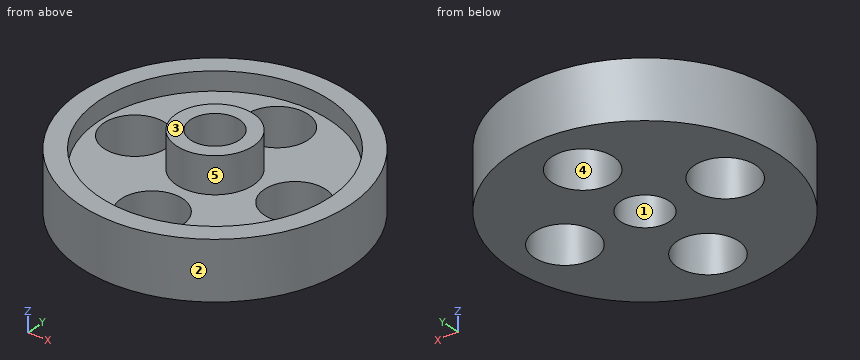
from build123d import *

# Parameters (mm, degrees)
F0_R     = 35.0012
F0_R_2   = 29.9974
F1_DEPTH = 15.0114
F0_R_3   = 8.001
F0_R_4   = 9.9949
F2_DEPTH = 10.16
F0_R_5   = 6.3373
F3_DEPTH = 19.5072


# Not quite as in the source:
# - a feature names something its author has since deleted; it is built from what else it names


with BuildPart() as f1:
    # F0 (on Top) → F1 (new body)
    with BuildSketch(Plane.XY):
        Circle(F0_R)
        Circle(F0_R_2, mode=Mode.SUBTRACT)
    extrude(amount=F1_DEPTH)

    # F0 (on Top) → F2 (join)
    with BuildSketch(Plane.XY):
        Circle(F0_R_2)
        with Locations((0.1067890262, -20.8610873669)):
            Circle(F0_R_3, mode=Mode.SUBTRACT)
        with Locations((20.7458101213, -0.0499814087)):
            Circle(F0_R_3, mode=Mode.SUBTRACT)
        with Locations((-20.7319166511, 0)):
            Circle(F0_R_3, mode=Mode.SUBTRACT)
        Circle(F0_R_4, mode=Mode.SUBTRACT)
        with Locations((0, 20.5026287585)):
            Circle(F0_R_3, mode=Mode.SUBTRACT)
    extrude(amount=F2_DEPTH)

    # F0 (on Top) → F3 (join)
    with BuildSketch(Plane.XY):
        Circle(F0_R_4)
        Circle(F0_R_5, mode=Mode.SUBTRACT)
    extrude(amount=F3_DEPTH)


solid = f1.part
Geometry: final body of the model. Coordinates: model frame, mm. Face numbers are marked on the shaded views. A direction names the side the tool comes from. Give positions to 0.01 mm unless a question says otherwise; leave off trailing zeros. Write each loop counter-clockwise with the first axis right and the second up, starting at its lowest first coordinate (ties: lowest second). Pieces come first, ordered by that corner, then holes.
(1) First-contact query: P1, Ø6, axis at x = -8.5, z = 12.5, coming from the -Y side; P2, Ø10, axis at y = 18, z = 13.5, coming from the -X side; P3, Ø2, axis at y = 7, z = 3, coming from the -X side. Flat tips, straight axial feed; report the tip coordinate or a pass-through.
(2) Cut plane D-D, the plane y = -4.5. Return loops of the section in (x, z).
(3) Ray query, line 1 (Y direction, x = 8.5, z = 11); line 2 (Y direction, x = 0, z = 13.2); line 3 (X direction, y = -4, z = 12). Return the intervals inside material, ascending.
(4) Mould query, pull axis Y, two halves, no side actions, for the marked faces 1, 2 and 3. Classes: released by +Y, released by -Y, zero draft, split by the parting line, or undercut.
(5) Cut plane A-A, the plane x = -14.5. Return loops of the section in (y, z).
(6) Access query for the marked faces 4 and 5. Directions: +Z, -Z, +X, -X, +Y, -Y. A direction counts if a zero-diameter tool reaches every point of the face in a straight line with its end or side. Return the directions, or none.
(7) Cut plane B-B, the plane x = 0. Return loops of the section in (y, z).
(8) Cut plane C-C, the plane y = -16.5. Return loops of the section in (x, z), then the cut area to 3 significant figures.
Values follow:
1. P1: stops at y = -34.57
1. P2: stops at x = -32.5
1. P3: stops at x = -34.48
2. outline: (-34.71, 0) - (-27.35, 0) - (-27.35, 10.16) - (-29.66, 10.16) - (-29.66, 15.01) - (-34.71, 15.01) - close; (-14.12, 0) - (-4.46, 0) - (-4.46, 19.51) - (-8.92, 19.51) - (-8.92, 10.16) - (-14.12, 10.16) - close; (4.46, 0) - (14.1, 0) - (14.1, 10.16) - (8.92, 10.16) - (8.92, 19.51) - (4.46, 19.51) - close; (27.4, 0) - (34.71, 0) - (34.71, 15.01) - (29.66, 15.01) - (29.66, 10.16) - (27.4, 10.16) - close
3. line 1: y = -33.95 to -28.77, -5.26 to 5.26, 28.77 to 33.95
3. line 2: y = -35 to -30, -9.99 to -6.34, 6.34 to 9.99, 30 to 35
3. line 3: x = -34.77 to -29.73, -9.16 to -4.92, 4.92 to 9.16, 29.73 to 34.77
4. face 1: undercut
4. face 2: split by the parting line
4. face 3: zero draft
5. outline: (-31.86, 0) - (-5.02, 0) - (-5.02, 10.16) - (-26.26, 10.16) - (-26.26, 15.01) - (-31.86, 15.01) - close; (5.02, 0) - (31.86, 0) - (31.86, 15.01) - (26.26, 15.01) - (26.26, 10.16) - (5.02, 10.16) - close
6. face 4: +Z, -Z
6. face 5: +Z
7. outline: (-35, 0) - (-28.86, 0) - (-28.86, 10.16) - (-30, 10.16) - (-30, 15.01) - (-35, 15.01) - close; (-12.86, 0) - (-6.34, 0) - (-6.34, 19.51) - (-9.99, 19.51) - (-9.99, 10.16) - (-12.86, 10.16) - close; (6.34, 0) - (12.5, 0) - (12.5, 10.16) - (9.99, 10.16) - (9.99, 19.51) - (6.34, 19.51) - close; (28.5, 0) - (35, 0) - (35, 15.01) - (30, 15.01) - (30, 10.16) - (28.5, 10.16) - close
8. outline: (-30.87, 0) - (-6.6, 0) - (-6.6, 10.16) - (-25.05, 10.16) - (-25.05, 15.01) - (-30.87, 15.01) - close; (6.81, 0) - (30.87, 0) - (30.87, 15.01) - (25.05, 15.01) - (25.05, 10.16) - (6.81, 10.16) - close
8. area: 547 mm2
